```python
from build123d import *

# Parameters (mm, degrees)
SKETCH1_R            = 16.4
BOSS_EXTRUDE7_DEPTH  = 2
BOSS_EXTRUDE9_DEPTH  = 2
CIRPATTERN3_COUNT    = 10
SKETCH8_R            = 15
CUT_EXTRUDE6_DEPTH   = 2
SKETCH9_R            = 0.219012447
BOSS_EXTRUDE10_DEPTH = 2
CIRPATTERN4_COUNT    = 10


with BuildPart() as part:
    # Sketch1 → Boss-Extrude7 (new body)
    with BuildSketch(Plane.XY):
        Circle(SKETCH1_R)
    boss_extrude7 = extrude(amount=BOSS_EXTRUDE7_DEPTH)

    # Sketch7 → Boss-Extrude9 (add)
    with BuildSketch(Plane(origin=(0, 0, 0), x_dir=(-1, 0, 0), z_dir=(0, 0, -1))):
        with BuildLine():
            Line((7.758615453, 23.765603006), (4.664676273, 15.722620496))
            ThreePointArc((4.664676273, 15.722620496), (2.678892521, 16.179726044), (0.651751249, 16.387044282))
            Line((0.651751249, 16.387044282), (0, 25))
            ThreePointArc((0, 25), (3.928099085, 24.689472201), (7.758615453, 23.765603006))
        make_face()
    boss_extrude9 = extrude(amount=-BOSS_EXTRUDE9_DEPTH)

    # CirPattern3: Boss-Extrude7, Boss-Extrude9 ×10 about axis
    cirpattern3_axis = Axis((0, 0, 0), (0, 0, 1))
    add([boss_extrude7.rotate(cirpattern3_axis, i * 360 / CIRPATTERN3_COUNT) for i in range(1, CIRPATTERN3_COUNT)])
    add([boss_extrude9.rotate(cirpattern3_axis, i * 360 / CIRPATTERN3_COUNT) for i in range(1, CIRPATTERN3_COUNT)])

    # Sketch8 → Cut-Extrude6 (cut)
    with BuildSketch(Plane.XY.offset(2)):
        Circle(SKETCH8_R)
    extrude(amount=-CUT_EXTRUDE6_DEPTH, mode=Mode.SUBTRACT)

    # Sketch9 → Boss-Extrude10 (add)
    with BuildSketch(Plane.XY.offset(2)):
        with Locations((-2.473101921, 15.544307771)):
            Circle(SKETCH9_R)
    boss_extrude10 = extrude(amount=BOSS_EXTRUDE10_DEPTH)

    # CirPattern4: Boss-Extrude10 ×10 about axis
    cirpattern4_axis = Axis((0, 0, 0), (0, 0, 1))
    for i in range(1, CIRPATTERN4_COUNT):
        add(boss_extrude10.rotate(cirpattern4_axis, i * 360 / CIRPATTERN4_COUNT))


solid = part.part
```
Work out the finished part from the listing and answer in its coordinate system (mm). A direction names the side the tool comes from. Give positions to 0.01 mm unless a question says otherwise; leave off trailing zeros. Order: outer loops, then holes, each group sorted by start corner. A loop starts at its lowest first (then second) coordinate and runs counter-clockwise, first axis right, second up.
1. Each of these flat-tipped pins is pushed along its axis until it touches: P1, Ø2, axis at y = -13, z = 1, coming from the -X side; P2, Ø1.5, axis at y = -8.5, z = 3.5, coming from the +X side. Where does it stop, or does it pass through?
Result sheet:
P1: stops at x = -21.93
P2: passes through
2. Section D-D, the plane y = 18.5 is taken. Determine the outline of the cut face in (x, z), and give its area (3 significant figures).
Result sheet:
outline: (-16.82, 0) - (-13.63, 0) - (-13.63, 2) - (-16.82, 2) - close; (-5.73, 0) - (-0.49, 0) - (-0.49, 2) - (-5.73, 2) - close; (6.28, 0) - (13.23, 0) - (13.23, 2) - (6.28, 2) - close
area: 30.8 mm2
3. For faces 4 (the flat face through (6.6, 19.7, 1)), 5 (the flat face through (-6.6, -19.7, 1)), 6 (the cylindrical face through (22.3, 11.3, 1)), 7 (the cylindrical face through (14.645, -7.382, 0.986)), 8 (the flat face through (-19.52, -6.69, 0.99)), determine the directions among +Z, -Z, +X, -X, +Y, -Y from which every point of the face is accessible in a straight line to the end or side of a thin tool.
Result sheet:
face 4: +Z, -Z, +Y
face 5: +Z, -Z, -Y
face 6: +Z, -Z, +X, +Y
face 7: +Z, -Z
face 8: +Z, -Z, -X
4. Section B-B, the plane y = -3.5 is taken. Determine the outline of the cut face in (x, z).
Result sheet:
outline: (-16.02, 0) - (-14.59, 0) - (-14.59, 2) - (-16.02, 2) - close; (14.59, 0) - (24.75, 0) - (24.75, 2) - (14.59, 2) - close
5. The mould has two halves that part along X. Classify faces 1 (the flat face through (-13, 8, 2)), 2 (the cylindrical face through (-17.651, 17.704, 0.986)), 3 (the cylindrical face through (-14.645, 7.382, 0.986)): released by +X, released by -X, zero draft, split by the parting line, or undercut.
Result sheet:
face 1: zero draft
face 2: released by -X
face 3: undercut
6. Straight lines are drawn through the part: L1, parallel to X at y = -20, z = 1.8; L2, parallel to Z at x = 5.5, y = -21.5; L3, parallel to X at y = 15.5, z = 3.15. For each, find the intervals that lie inside material, in ascending order.
Result sheet:
L1: x = -14.5 to -6.68, 0.38 to 6.31, 14.56 to 15
L2: z = 0 to 2
L3: x = -2.69 to -2.26
7. Section C-C, the plane z = 3.05 is taken. Give the number of separate pieces and of enclosed holes in the cut face, and give its area (3 significant figures).
Result sheet:
separate pieces: 10
enclosed holes: 0
area: 1.51 mm2
8. Section A-A, the plane x = 18 is taken. Determine the outline of the cut face in (y, z), and give its area (3 significant figures).
Result sheet:
outline: (-17.35, 0) - (-13.21, 0) - (-13.21, 2) - (-17.35, 2) - close; (-5.35, 0) - (-0.34, 0) - (-0.34, 2) - (-5.35, 2) - close; (6.32, 0) - (12.93, 0) - (12.93, 2) - (6.32, 2) - close
area: 31.5 mm2
